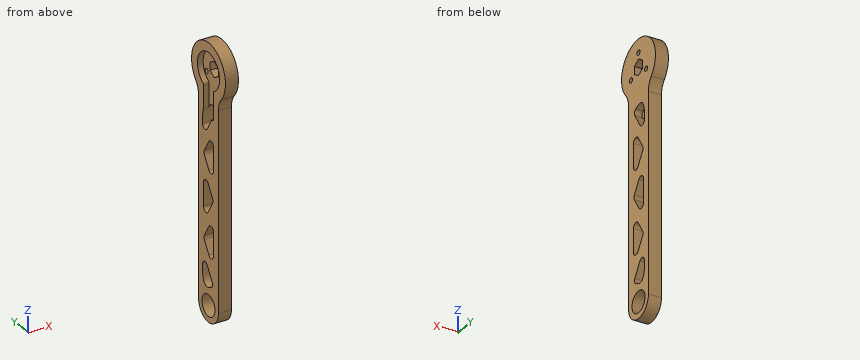
```python
from build123d import *

# Parameters (mm, degrees)
SKETCH_1_R          = 6.55
EXTRUDE_1_DEPTH     = 8
CUT_EXTRUDE_1_DEPTH = 3.5
SKETCH_3_R          = 1.55
CUT_EXTRUDE_2_DEPTH = 5.5000001


with BuildPart() as part:
    # 草图1 → 凸台-拉伸1 (new body)
    with BuildSketch(Plane(origin=(-4, 0, 0), x_dir=(0, -1, 0), z_dir=(-1, 0, 0))):
        with BuildLine():
            Line((-10, -18.894443628), (-10, -140))
            ThreePointArc((-10, -140), (0, -150), (10, -140))
            Line((10, -140), (10, -18.894443628))
            ThreePointArc((10, -18.894443628), (10.74741409, -14.725593625), (12.896551724, -11.076053161))
            ThreePointArc((12.896551724, -11.076053161), (0, 17), (-12.896551724, -11.076053161))
            ThreePointArc((-12.896551724, -11.076053161), (-10.74741409, -14.725593625), (-10, -18.894443628))
        make_face()
        with Locations((0, -140)):
            Circle(SKETCH_1_R, mode=Mode.SUBTRACT)
        with BuildLine():
            Line((-4.168179012, -99.797532142), (0.381550311, -92.536811957))
            ThreePointArc((0.381550311, -92.536811957), (3.190606899, -91.461560083), (5, -93.864279815))
            Line((5, -93.864279815), (5, -108.385720185))
            ThreePointArc((5, -108.385720185), (3.190606899, -110.788439917), (0.381550311, -109.713188043))
            Line((0.381550311, -109.713188043), (-4.168179012, -102.452467858))
            ThreePointArc((-4.168179012, -102.452467858), (-4.549729323, -101.125), (-4.168179012, -99.797532142))
        make_face(mode=Mode.SUBTRACT)
        with BuildLine():
            Line((-1.347932676, -116.369603301), (3.683273316, -124.398691695))
            ThreePointArc((3.683273316, -124.398691695), (3.98786354, -126.341689874), (2.792876182, -127.903746961))
            add(Edge.make_bspline(
                [(2.792876182, -127.903746961), (-2.877603269, -131.101619406), (-5.985402229, -127.808170374), (-6.076762251, -119.793304589), (-5.963124704, -117.569487096)],
                knots=[0.005408839, 0.005408839, 0.005408839, 0.005408839, 0.693539789, 0.980498212, 0.980498212, 0.980498212, 0.980498212], degree=3))
            ThreePointArc((-5.963124704, -117.569487096), (-4.09543452, -115.277506448), (-1.347932676, -116.369603301))
        make_face(mode=Mode.SUBTRACT)
        with BuildLine():
            Line((0.381550311, -58.963188043), (-4.168179012, -51.702467858))
            ThreePointArc((-4.168179012, -51.702467858), (-4.549729323, -50.375), (-4.168179012, -49.047532142))
            Line((-4.168179012, -49.047532142), (0.381550311, -41.786811957))
            ThreePointArc((0.381550311, -41.786811957), (3.190606899, -40.711560083), (5, -43.114279815))
            Line((5, -43.114279815), (5, -57.635720185))
            ThreePointArc((5, -57.635720185), (3.190606899, -60.038439917), (0.381550311, -58.963188043))
        make_face(mode=Mode.SUBTRACT)
        with BuildLine():
            Line((3.683273317, -27.101308304), (-1.347932676, -35.130396699))
            ThreePointArc((-1.347932676, -35.130396699), (-4.095434519, -36.222493552), (-5.963124704, -33.930512906))
            add(Edge.make_bspline(
                [(-5.963124704, -33.930512906), (-6.076762251, -31.706695412), (-5.98540223, -23.691829624), (-2.877603269, -20.398380591), (2.792876182, -23.596253037)],
                knots=[0.005408839, 0.005408839, 0.005408839, 0.005408839, 0.292367263, 0.980498213, 0.980498213, 0.980498213, 0.980498213], degree=3))
            ThreePointArc((2.792876182, -23.596253037), (3.987863541, -25.158310124), (3.683273317, -27.101308304))
        make_face(mode=Mode.SUBTRACT)
        with BuildLine():
            Line((4.168179012, -77.077467858), (-0.381550311, -84.338188043))
            ThreePointArc((-0.381550311, -84.338188043), (-3.190606899, -85.413439917), (-5, -83.010720185))
            Line((-5, -83.010720185), (-5, -68.489279815))
            ThreePointArc((-5, -68.489279815), (-3.190606899, -66.086560083), (-0.381550311, -67.161811957))
            Line((-0.381550311, -67.161811957), (4.168179012, -74.422532142))
            ThreePointArc((4.168179012, -74.422532142), (4.549729323, -75.75), (4.168179012, -77.077467858))
        make_face(mode=Mode.SUBTRACT)
    extrude(amount=-EXTRUDE_1_DEPTH)

    # 草图2 → 切除-拉伸1 (cut)
    with BuildSketch(Plane.ZY.offset(4)):
        with BuildLine():
            Line((-23.794604197, 5), (-27.625420737, 5))
            Line((-27.625420737, 5), (-27.625420737, -4.039591784))
            ThreePointArc((-27.625420737, -4.039591784), (-27.344123683, -4.718702946), (-26.665012521, -5))
            Line((-26.665012521, -5), (-23.794604197, -5))
            Line((-23.794604197, -5), (-10.507616285, -5))
            ThreePointArc((-10.507616285, -5), (-10.005554421, -5.135168291), (-9.639218245, -5.504132231))
            ThreePointArc((-9.639218245, -5.504132231), (11.1, 0), (-9.639218245, 5.504132231))
            ThreePointArc((-9.639218245, 5.504132231), (-10.005554421, 5.135168291), (-10.507616285, 5))
            Line((-10.507616285, 5), (-23.794604197, 5))
        make_face()
    extrude(amount=-CUT_EXTRUDE_1_DEPTH, mode=Mode.SUBTRACT)

    # 草图3 → 切除-拉伸2 (cut, through all)
    with BuildSketch(Plane.ZY.offset(0.5)):
        with Locations((-4.375, 7.577722283)):
            Circle(SKETCH_3_R)
        with Locations((-4.375, -7.577722283)):
            Circle(SKETCH_3_R)
        with Locations((8.75, 0)):
            Circle(SKETCH_3_R)
        Polygon((4.907477288, 0), (2.453738644, 4.25), (-2.453738644, 4.25), (-4.907477288, 0), (-2.453738644, -4.25), (2.453738644, -4.25), align=None)
    extrude(amount=-CUT_EXTRUDE_2_DEPTH, mode=Mode.SUBTRACT)


solid = part.part
```
Build history of the part. All positions in model axes, mm. Coordinates: 2 decimals unless noted, no trailing zeros. Order: outer loops, then holes, each group sorted by start corner. A loop starts at its lowest first (then second) coordinate and runs counter-clockwise, first axis right, second up. Notation, with made-up numbers: (33.25, 79.5) -> (51.25, 79.5) arc R28 cw to (51.25, 107.5) -> close; hole circle Ø1 at (-21, 75). An arc over 180 degrees is marked (long way). Answer in a Markdown table with one row per item. Add a question column.
Q1. Wall check: line 1 along Y through (x, z) = (0.5, -99); line 2 along Z through (x, y) = (-2, -9); line 3 along Y through (x, z) = (-3, -119.5). Give the ranges that are in metal, low to high. Write a range as [from, to].
Q2. Band-saw the part on C-C, the plane y = 15. List the corners of the cut face in (x, z).
Q3. Drop flat-ended pins along their axis: pin 1 (2 mm diameter, centred on x = -1, z = -101.5, fed in from +Y); pin 2 (4 mm diameter, centred on x = -3, z = -16, fed in from +Y); pin 3 (2.5 mm diameter, centred on x = 0, z = -78.5, fed in from -Y); pin 4 (10.5 mm diameter, centred on y = 0, z = -140, fed in from +X). Give the stop position or say it passes through.
Q4. Band-saw the part on B-B, the plane z = -135. List the corners of the cut face in (x, y), then the cut area to 3 significant figures.
Q5. Band-saw the part on A-A, the plane z = 0. List the corners of the cut face in (x, y), then the cut area to 3 significant figures.
Answers follow:
| question | item | result |
|---|---|---|
| 1 | line 1 | [-10, -5], [3.67, 10] |
| 1 | line 2 | [-144.36, -6.5], [6.5, 14.42] |
| 1 | line 3 | [-10, -0.61], [6.02, 10] |
| 2 | outline | (-4, -8) -> (4, -8) -> (4, 8) -> (-4, 8) -> close |
| 3 | pin 1 | y = 10 |
| 3 | pin 2 | y = 11.04 |
| 3 | pin 3 | y = -10 |
| 3 | pin 4 | through |
| 4 | outline | (-4, -10) -> (4, -10) -> (4, -4.23) -> (-4, -4.23) -> close; (-4, 4.23) -> (4, 4.23) -> (4, 10) -> (-4, 10) -> close |
| 4 | area | 92.3 mm^2 |
| 5 | outline | (-4, -17) -> (4, -17) -> (4, -4.25) -> (-0.5, -4.25) -> (-0.5, -11.1) -> (-4, -11.1) -> close; (-4, 11.1) -> (-0.5, 11.1) -> (-0.5, 4.25) -> (4, 4.25) -> (4, 17) -> (-4, 17) -> close |
| 5 | area | 156 mm^2 |
